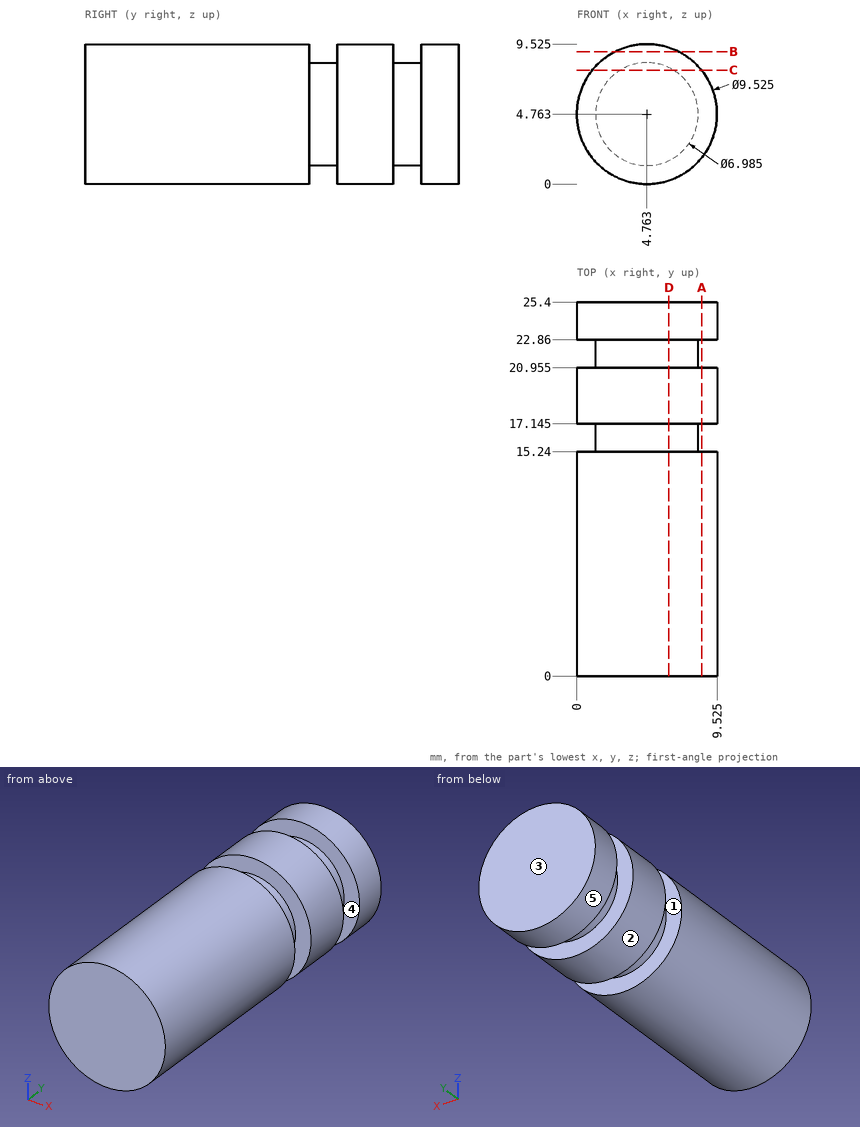
Print and shaded views of the part. All mm, measured from the part's lowest x, y and z. A direction names the side the tool comes from. Coordinates: 2 decimals unless noted, no trailing zeros. Order: outer loops, then holes, each group sorted by start corner. A loop starts at its lowest first (then second) coordinate and runs counter-clockwise, first axis right, second up. Notation, with made-up numbers: (-35, 48.25) - (-28, 48.25) arc R17 cw to (-28, 66.25) - close; hole circle Ø7 at (51, -24). An arc over 180 degrees is marked (long way). Return JSON: item names as keys, results as strings. Group by question number.
Item 1: Drill centre lines: probe 1 along Y at (x, z) = (0.75, 6.25) (1 decimal); probe 2 along X at (y, z) = (17.5, 8) (1 decimal); probe 3 along X at (y, z) = (1.75, 5) (1 decimal). Where is each one in solid material? Low to high. Write a range as from..to.
Item 2: Cut at D-D (x = 6.25). List the corners of the cut face in (y, z) (1 decimal).
Item 3: Cut at B-B (z = 9). List the corners of the cut face in (x, y) (1 decimal).
Item 4: Pull direction Y, two halves, no side cores. Call the marked faces 3, 4 and 5: pulls with the +Y half, pulls with the -Y half, needs draft (parallel to the pull), parting line crosses it, or undercut.
Item 5: Cut at C-C (z = 7.75). List the corners of the cut face in (x, y) (1 decimal).
Item 6: Pin check, flat tips, straight feed: pin 1 (3 mm diameter, centred on x = 7, y = 12.5, fed in from +Z); pin 2 (3 mm diameter, centred on x = 6, z = 3.5, fed in from -Y); pin 3 (4 mm diameter, centred on x = 7.5, y = 15, fed in from -Z); pin 4 (2 mm diameter, centred on x = 2.5, y = 17, fed in from -Z). Stop position of each tip, or through.
Item 7: Cut at A-A (x = 8.5). List the corners of the cut face in (y, z) (1 decimal).
Item 8: Which spindle directions (+Z, -Z, +X, -X, +Y, -Y) get a long thin tool onto all of the face, cutting with end or side? Do the marked faces 1 and 2. Say none if no direction does.
Check values:
{
 "1": {"probe 1": "y = 0..15.2, 17.1..21, 22.9..25.4", "probe 2": "x = 1.3..8.3", "probe 3": "x = 0..9.5"},
 "2": {"outline": "(0, 0.2) - (15.2, 0.2) - (15.2, 1.6) - (17.1, 1.6) - (17.1, 0.2) - (21, 0.2) - (21, 1.6) - (22.9, 1.6) - (22.9, 0.2) - (25.4, 0.2) - (25.4, 9.3) - (22.9, 9.3) - (22.9, 7.9) - (21, 7.9) - (21, 9.3) - (17.1, 9.3) - (17.1, 7.9) - (15.2, 7.9) - (15.2, 9.3) - (0, 9.3) - close"},
 "3": {"outline": "(2.6, 0) - (6.9, 0) - (6.9, 15.2) - (2.6, 15.2) - close; (2.6, 17.1) - (6.9, 17.1) - (6.9, 21) - (2.6, 21) - close; (2.6, 22.9) - (6.9, 22.9) - (6.9, 25.4) - (2.6, 25.4) - close"},
 "4": {"face 3": "pulls with the +Y half", "face 4": "undercut", "face 5": "needs draft"},
 "5": {"outline": "(1.1, 0) - (8.5, 0) - (8.5, 15.2) - (6.6, 15.2) - (6.6, 17.1) - (8.5, 17.1) - (8.5, 21) - (6.6, 21) - (6.6, 22.9) - (8.5, 22.9) - (8.5, 25.4) - (1.1, 25.4) - (1.1, 22.9) - (3, 22.9) - (3, 21) - (1.1, 21) - (1.1, 17.1) - (3, 17.1) - (3, 15.2) - (1.1, 15.2) - close"},
 "6": {"pin 1": "stops at z = 9.47", "pin 2": "stops at y = 0", "pin 3": "stops at z = 0.06", "pin 4": "stops at z = 0.17"},
 "7": {"outline": "(0, 1.8) - (15.2, 1.8) - (15.2, 7.7) - (0, 7.7) - close; (17.1, 1.8) - (21, 1.8) - (21, 7.7) - (17.1, 7.7) - close; (22.9, 1.8) - (25.4, 1.8) - (25.4, 7.7) - (22.9, 7.7) - close"},
 "8": {"face 1": "none", "face 2": "+Y, -Y"}
}
